from build123d import *

# Parameters (mm, degrees)
CROQUIS1_R              = 7.5
CROQUIS1_R_2            = 1.85
SALIENTE_EXTRUIR1_DEPTH = 25
CROQUIS2_R              = 6.5
CORTAR_EXTRUIR1_DEPTH   = 7.5
CROQUIS3_R              = 9
SALIENTE_EXTRUIR2_DEPTH = 2.5
CROQUIS4_R              = 3.1
CORTAR_EXTRUIR2_DEPTH   = 3.5
CROQUIS5_R              = 3.075
CORTAR_EXTRUIR3_DEPTH   = 4
REDONDEO1_R             = 0.5
CROQUIS6_R              = 1.75
CORTAR_EXTRUIR4_DEPTH   = 3.4


with BuildPart() as part:
    # Croquis1 → Saliente-Extruir1 (new body)
    with BuildSketch(Plane.XY):
        Circle(CROQUIS1_R)
        Circle(CROQUIS1_R_2, mode=Mode.SUBTRACT)
    extrude(amount=SALIENTE_EXTRUIR1_DEPTH)

    # Croquis2 → Cortar-Extruir1 (cut, symmetric)
    with BuildSketch(Plane.XY.offset(12.5)):
        Circle(CROQUIS2_R)
    extrude(amount=CORTAR_EXTRUIR1_DEPTH, both=True, mode=Mode.SUBTRACT)

    # Croquis3 → Saliente-Extruir2 (add)
    with BuildSketch(Plane(origin=(0, 0, 0), x_dir=(-1, 0, 0), z_dir=(0, 0, -1))):
        Circle(CROQUIS3_R)
    extrude(amount=SALIENTE_EXTRUIR2_DEPTH)

    # Croquis4 → Cortar-Extruir2 (cut)
    with BuildSketch(Plane.XY.offset(25)):
        Circle(CROQUIS4_R)
    extrude(amount=-CORTAR_EXTRUIR2_DEPTH, mode=Mode.SUBTRACT)

    # Croquis5 → Cortar-Extruir3 (cut)
    with BuildSketch(Plane(origin=(0, 0, -2.5), x_dir=(-1, 0, 0), z_dir=(0, 0, -1))):
        Circle(CROQUIS5_R)
    extrude(amount=-CORTAR_EXTRUIR3_DEPTH, mode=Mode.SUBTRACT)

    # Redondeo1
    redondeo1_edges = [part.edges().sort_by_distance(p)[0] for p in [
        (3.075, 0, -2.5),
    ]]
    fillet(redondeo1_edges, radius=REDONDEO1_R)

    # Croquis6 → Cortar-Extruir4 (cut)
    with BuildSketch(Plane(origin=(0, 0, -2.5), x_dir=(-1, 0, 0), z_dir=(0, 0, -1))):
        with Locations((-5.5, 0)):
            Circle(CROQUIS6_R)
        with Locations(Location((5.5, 0, 0), (0, 0, 180))):
            Circle(CROQUIS6_R)
    extrude(amount=-CORTAR_EXTRUIR4_DEPTH, mode=Mode.SUBTRACT)


solid = part.part
Check sheet for the modelled part. Datum: model origin and axes. Units: mm. A direction names the side the tool comes from. Give positions to 0.01 mm unless a question says otherwise; leave off trailing zeros. Loops run counter-clockwise (first coordinate to the right, second up) from the corner with the lowest first, then second, coordinate; pieces in that order, holes last. Notation, with made-up numbers: M 38.5,28.5 L 74.5,28.5 A26 cw 74.5,61.5 Z; hole C -3,-20 d2. An arc over 180 degrees is marked long. Answer as a JSON object with one key per item and string values. Group by question number.
Q1. Cross-section at C-C on z = 20.75. Record the cut outline in (x, y).
Q2. Release check for a two-part mould opening along Y. For faces 4 (the cylindrical face through (1.172, 8.923, -1.232)), 5 (the flat face through (2, 7.4, 0)), 6 (the cylindrical face through (-0.401, -1.806, 3.226)) record: released by +Y, released by -Y, zero draft, split by the parting line, or undercut.
Q3. Cross-section at B-B on y = 5.5. Record the cut outline in (x, z).
Q4. Material ranges on line 1 along Z through (x, y) = (1.5, -2.25); line 2 along Z through (x, y) = (2.75, -5.25); line 3 along Y through (x, z) = (0, -1.1) (3 decimals), recorded low to high. Write a range as [from, to].
Q5. Access from +Z, -Z, +X, -X, +Y, -Y to the whole of each face (thin tool, end or side, straight path). Record for faces 1 (the cylindrical face through (0.67, -3, -0.27)), 2 (the flat face through (1, 2, 20)), 3 (the cylindrical face through (1.43, -2.75, 23.27)).
Q6. Cross-section at D-D on x = -6. Record the cut outline in (y, z), then the cut area to 3 significant figures.
Q7. Go/stop test with flat-tipped pins: P1, Ø5, axis at x = 2, z = 3, coming from the +Y side; P2, Ø2, axis at x = 0, y = 0, coming from the -Z side; P3, Ø5.5, axis at x = 0, y = 0, coming from the +Z side; P4, Ø6, axis at x = 0, y = 0, coming from the -Z side. Record where each tip stops, or that it passes through.
Evaluation:
{
 "1": {"outline": "C 0,0 d15; hole C 0,0 d3.7"},
 "2": {"face 4": "split by the parting line", "face 5": "zero draft", "face 6": "undercut"},
 "3": {"outline": "M -7.12,-2.5 L 7.12,-2.5 L 7.12,0 L 5.1,0 L 5.1,25 L -5.1,25 L -5.1,0 L -7.12,0 Z; hole M -3.46,5 L 3.46,5 L 3.46,20 L -3.46,20 Z"},
 "4": {"line 1": "z = [1.5, 5], [20, 21.5]", "line 2": "z = [-2.5, 5], [20, 25]", "line 3": "y = [-9, -3.075], [3.075, 9]"},
 "5": {"face 1": "-Z", "face 2": "none", "face 3": "+Z"},
 "6": {"outline": "M -6.71,-2.5 L -1.68,-2.5 L -1.68,0.9 L 1.68,0.9 L 1.68,-2.5 L 6.71,-2.5 L 6.71,0 L 4.5,0 L 4.5,25 L -4.5,25 L -4.5,0 L -6.71,0 Z; hole M -2.5,5 L 2.5,5 L 2.5,20 L -2.5,20 Z", "area": "172 mm2"},
 "7": {"P1": "stops at y = 7.5", "P2": "passes through", "P3": "stops at z = 21.5", "P4": "stops at z = 1.5"}
}
